Geometry check sheet. Reference: the model listing, model coordinates, mm. A direction names the side the tool comes from. Coordinates: 2 decimals unless noted, no trailing zeros. Write each loop counter-clockwise with the first axis right and the second up, starting at its lowest first coordinate (ties: lowest second). Pieces come first, ordered by that corner, then holes. Notation, with made-up numbers: M -10,24 L 41,24 A12 cw 41,29 Z; hole C 60,24 d4. An arc over 180 degrees is marked long. Write each question's results on one line, items separated by ' | '.
```python
from build123d import *

# Parameters (mm, degrees)
SKETCH1_W           = 10
SKETCH1_H           = 10
BOSS_EXTRUDE3_DEPTH = 3
SKETCH5_W           = 1
SKETCH5_H           = 1
BOSS_EXTRUDE4_DEPTH = 10.4
SKETCH6_W           = 1
SKETCH6_H           = 1.9
BOSS_EXTRUDE5_DEPTH = 12.5


with BuildPart() as part:
    # Sketch1 → Boss-Extrude3 (new body)
    with BuildSketch(Plane.XY):
        Rectangle(SKETCH1_W, SKETCH1_H)
    extrude(amount=-BOSS_EXTRUDE3_DEPTH)

    # Sketch5 → Boss-Extrude4 (add)
    with BuildSketch(Plane.XY):
        Rectangle(SKETCH5_W, SKETCH5_H)
    extrude(amount=BOSS_EXTRUDE4_DEPTH)

    # Sketch6 → Boss-Extrude5 (add)
    with BuildSketch(Plane(origin=(0, 0.5, 0), x_dir=(1, 0, 0), z_dir=(0, 1, 0))):
        with Locations((0, -9.45)):
            Rectangle(SKETCH6_W, SKETCH6_H)
    extrude(amount=-BOSS_EXTRUDE5_DEPTH)


solid = part.part
```
Q1. Access from +Z, -Z, +X, -X, +Y, -Y to the whole of each face (thin tool, end or side, straight path). Record for faces 1 (the flat face through (0, -6, 8.5)), 2 (the flat face through (-0.5, -4, 9)), 3 (the flat face through (0.5, -4, 9)), 4 (the flat face through (0, 0.5, 5)).
Geometry check:
face 1: +X, -X, -Y | face 2: +Z, -X, +Y, -Y | face 3: +Z, +X, +Y, -Y | face 4: +Z, +X, -X, +Y
Q2. Sectioned sample at A-A on y = -3.5. Record the cut outline in (x, z).
Geometry check:
outline: M -5,-3 L 5,-3 L 5,0 L -5,0 Z; M -0.5,8.5 L 0.5,8.5 L 0.5,10.4 L -0.5,10.4 Z
Q3. Sectioned sample at B-B on x = 0.25. Record the cut outline in (y, z), and give its area (4 significant figures).
Geometry check:
outline: M -12,8.5 L -0.5,8.5 L -0.5,0 L -5,0 L -5,-3 L 5,-3 L 5,0 L 0.5,0 L 0.5,10.4 L -12,10.4 Z | area: 62.25 mm2
Q4. Depth check by flat-ended pin: P1, Ø4, axis at y = -7.5, z = 8.5, coming from the -X side; P2, Ø5, axis at x = 3.5, z = 3, coming from the -Y side; P3, Ø3.5, axis at x = 0.5, z = -1, coming from the -Y side; P4, Ø0.5, axis at x = 0, y = -6.5, coming from the -Z side. Enter the tip coordinate at first touch or a pass-through.
Geometry check:
P1: stops at x = -0.5 | P2: passes through | P3: stops at y = -5 | P4: stops at z = 8.5
Q5. Sectioned sample at C-C on z = -0.75. Record the cut outline in (x, y).
Geometry check:
outline: M -5,-5 L 5,-5 L 5,5 L -5,5 Z
Q6. Mould release check, pull along Z, two halves, no side actions. Record for faces 5 (the flat face through (0, -5, -1)), 6 (the flat face through (0, 0, -3)), 7 (the flat face through (0, -0.5, 4)): pulls with the +Z half, pulls with the -Z half, needs draft (parallel to the pull), parting line crosses it, or undercut.
Geometry check:
face 5: needs draft | face 6: pulls with the -Z half | face 7: undercut
Q7. Scan lines: probe 1 along Z at (x, y) = (-1.5, -4); probe 2 along Z at (x, y) = (0.25, -6); probe 3 along Y at (x, z) = (-0.75, -2.5). Record each from-to range of solid material in increasing order.
Geometry check:
probe 1: z = -3 to 0 | probe 2: z = 8.5 to 10.4 | probe 3: y = -5 to 5
Q8. Sectioned sample at D-D on y = 0.25. Record the cut outline in (x, z).
Geometry check:
outline: M -5,-3 L 5,-3 L 5,0 L 0.5,0 L 0.5,10.4 L -0.5,10.4 L -0.5,0 L -5,0 Z
